Geometry: final body of the model. Coordinates: model frame, mm. A direction names the side the tool comes from. Round coordinates to 2 decimals unless told otherwise and drop trailing zeros. Loops run counter-clockwise (first coordinate to the right, second up) from the corner with the lowest first, then second, coordinate; pieces in that order, holes last. Notation, with made-up numbers: (70.25, 77) - (108.25, 77) arc R19 cw to (108.25, 88) - close; hole circle Ø2 at (59.25, -32.5). An arc over 180 degrees is marked (long way). Answer as a JSON object with one key per item and string values. Group by question number.
Item 1: Draft query along Y for faces 4 (the face through (164.9, 76.6, -0.4)), 5 (the face through (165, -1, -76.2)), 6 (the face through (241.5, -88.7, -38.3)), 7 (the face through (208.1, 3.7, -38.3)). Return one class per face: released by +Y, released by -Y, zero draft, split by the parting line, or undercut.
Item 2: Section C-C (z = -37.5). Return the cut outline in (x, y).
Item 3: Line query: line 1 (X direction, y = 65, z = -41); line 2 (Z direction, x = 197.5, y = 16.5); line 3 (X direction, y = -28, z = -40.5). Output: solid intervals per line, ascending.
Item 4: First-contact query: pin 1 (6 mm diameter, centred on y = -21.5, z = -6, fed in from -X); pin 2 (12 mm diameter, centred on y = 79, z = -14.5, fed in from +X); pin 3 (19 mm diameter, centred on x = 212.82, y = 0, fed in from +Z). Flat tips, straight axial feed; report the tip coordinate or a pass-through.
Item 5: Section A-A (y = 0). Return the cut outline in (x, z).
Item 6: Section D-D (x = 174.5). Return the cut outline in (y, z), plus the area to 3 significant figures.
Item 7: Reachability of faces 1 (the face through (177.8, -1, -63)), 2 (the face through (75.13, -2.75, -12.4)), 3 (the face through (224, -1, -25.4)) from +Z, -Z, +X, -X, +Y, -Y: full face, straight path, thin tool, end or side. Return the list, or none.
Item 8: Section B-B (y = -87.5). Return the cut outline in (x, z), plus the area to 3 significant figures.
```python
from build123d import *

# Parameters (mm, degrees)
F0_R     = 12.7
F1_DEPTH = 152.4
F2_W     = 203.2
F2_H     = 101.6
F3_DEPTH = 25.4
F4_SIZE  = 50.8
F5_W     = 203.2
F5_H     = 25.4
F6_DEPTH = 76.2
F7_SIZE  = 25.4
F8_R     = 6
F9_DEPTH = 76.201


with BuildPart() as f1:
    # F0 (on Right) → F1 (new body)
    with BuildSketch(Plane.YZ):
        Circle(F0_R)
    extrude(amount=F1_DEPTH)

    # F2 (on face) → F3 (join)
    with BuildSketch(Plane.YZ.offset(152.4)):
        with Locations((0, -25.4)):
            Rectangle(F2_W, F2_H)
    extrude(amount=F3_DEPTH)

    # F4
    f4_edges = [f1.edges().sort_by_distance(p)[0] for p in [
        (165.1, 101.6, 25.4),
        (165.1, -101.6, 25.4),
    ]]
    chamfer(f4_edges, length=F4_SIZE)

    # F5 (on face) → F6 (join)
    with BuildSketch(Plane.YZ.offset(177.8)):
        with Locations((0, -38.1)):
            Rectangle(F5_W, F5_H)
    extrude(amount=F6_DEPTH)

    # F7
    f7_edges = [f1.edges().sort_by_distance(p)[0] for p in [
        (254, -101.6, -38.1),
        (254, 101.6, -38.1),
    ]]
    chamfer(f7_edges, length=F7_SIZE)

    # F8 (on face) → F9 (cut, through all)
    with BuildSketch(Plane(origin=(0, 0, -50.8), x_dir=(1, 0, 0), z_dir=(0, 0, -1))):
        with Locations((219.188081, 65)):
            Circle(F8_R)
        with Locations((212.821616, 0)):
            Circle(F8_R)
        with Locations((219.188081, -65)):
            Circle(F8_R)
    extrude(amount=-F9_DEPTH, mode=Mode.SUBTRACT)


solid = f1.part
```
Values:
{
 "1": {"face 4": "released by +Y", "face 5": "zero draft", "face 6": "released by -Y", "face 7": "undercut"},
 "2": {"outline": "(152.4, -101.6) - (228.6, -101.6) - (254, -76.2) - (254, 76.2) - (228.6, 101.6) - (152.4, 101.6) - close; hole circle Ø12 at (212.82, 0); hole circle Ø12 at (219.19, -65); hole circle Ø12 at (219.19, 65)"},
 "3": {"line 1": "x = 152.4 to 213.19, 225.19 to 254", "line 2": "z = -50.8 to -25.4", "line 3": "x = 152.4 to 254"},
 "4": {"pin 1": "stops at x = 152.4", "pin 2": "stops at x = 177.8", "pin 3": "stops at z = -25.4"},
 "5": {"outline": "(0, -12.7) - (152.4, -12.7) - (152.4, -76.2) - (177.8, -76.2) - (177.8, -50.8) - (206.82, -50.8) - (206.82, -25.4) - (177.8, -25.4) - (177.8, 25.4) - (152.4, 25.4) - (152.4, 12.7) - (0, 12.7) - close; (218.82, -50.8) - (254, -50.8) - (254, -25.4) - (218.82, -25.4) - close"},
 "6": {"outline": "(-101.6, -76.2) - (101.6, -76.2) - (101.6, -25.4) - (50.8, 25.4) - (-50.8, 25.4) - (-101.6, -25.4) - close", "area": "18,100 mm^2"},
 "7": {"face 1": "-Z, +X, +Y, -Y", "face 2": "-X", "face 3": "+Z, +X, +Y, -Y"},
 "8": {"outline": "(152.4, -76.2) - (177.8, -76.2) - (177.8, -50.8) - (242.7, -50.8) - (242.7, -25.4) - (177.8, -25.4) - (177.8, -11.3) - (152.4, -11.3) - close", "area": "3,300 mm^2"}
}
